Geometry: final body of the model. Coordinates: model frame, mm. A direction names the side the tool comes from. Give positions to 0.01 mm unless a question says otherwise; leave off trailing zeros. Loops run counter-clockwise (first coordinate to the right, second up) from the corner with the lowest first, then second, coordinate; pieces in that order, holes last.
Solid Edge part; units mm, degrees
sketch "Sketch1" plane through (0, 0, 0) normal (0, -1, 0) x (1, 0, 0)
  line L0 (-20.5, 32.9403) -> (20.5, 32.9403)
  line L1 (20.5, 32.9403) -> (20.5, 22.9403)
  line L2 (20.5, 22.9403) -> (28.5, 22.9403)
  line L3 (28.5, 22.9403) -> (28.5, 20.9403)
  line L4 (28.5, 20.9403) -> (20.5, 20.9403)
  line L5 (20.5, 20.9403) -> (20.5, -5.0597)
  line L6 (-20.5, -5.0597) -> (20.5, -5.0597)
  line L7 (-20.5, 20.9403) -> (-20.5, -5.0597)
  line L8 (-28.5, 20.9403) -> (-20.5, 20.9403)
  line L9 (-28.5, 22.9403) -> (-28.5, 20.9403)
  line L10 (-20.5, 22.9403) -> (-28.5, 22.9403)
  line L11 (-20.5, 32.9403) -> (-20.5, 22.9403)
  dimension "D1" = 20.5
  dimension "D2" = 20.5
  dimension "D3" = 28.5
  dimension "D4" = 20.5
  dimension "D5" = 28.5
extrude "Protrusion1" add sketch "Sketch1" along normal mid plane 21
sketch "Sketch2" plane through (0, 0, 32.9403) normal (0, 0, 1) x (1, 0, 0)
  circle A0 centre (-10.5, 0) radius 3
extrude "ProtrusiónExtruida_2" add sketch "Sketch2" along normal mid plane 4
Item 1: Section query D-D on y = 0. Return loops of the section in (x, z), plus the area to 3 significant figures.
Values follow:
outline: (-28.5, 20.94) - (-20.5, 20.94) - (-20.5, -5.06) - (20.5, -5.06) - (20.5, 20.94) - (28.5, 20.94) - (28.5, 22.94) - (20.5, 22.94) - (20.5, 32.94) - (-7.5, 32.94) - (-7.5, 34.94) - (-13.5, 34.94) - (-13.5, 32.94) - (-20.5, 32.94) - (-20.5, 22.94) - (-28.5, 22.94) - close
area: 1,600 mm2
Item 2: Section query A-A on x = -10.5. Return loops of the section in (y, z).
Values follow:
outline: (-10.5, -5.06) - (10.5, -5.06) - (10.5, 32.94) - (3, 32.94) - (3, 34.94) - (-3, 34.94) - (-3, 32.94) - (-10.5, 32.94) - close
Item 3: Set-up query: faces 1 (the face through (-12.9, 1.8, 33.9)), 2 (the face through (-25, 0, 20.94)), 3 (the face through (-20.5, 0, 28)), 4 (the face through (25, 0, 20.94)). Return all of +Z, -Z, +X, -X, +Y, -Y with unobstructed straight access to the full face (end or side cutting, diameter ignored); none if empty.
Values follow:
face 1: +Z
face 2: -Z, -X, +Y, -Y
face 3: +Z, -X, +Y, -Y
face 4: -Z, +X, +Y, -Y
Item 4: Section query C-C on z = 1. Return loops of the section in (x, y), plus the area to 3 significant figures.
Values follow:
outline: (-20.5, -10.5) - (20.5, -10.5) - (20.5, 10.5) - (-20.5, 10.5) - close
area: 861 mm2
Item 5: Ray query, probe 1 along Z at (x, y) = (9, -1.5); probe 2 along X at (y, z) = (-8, 2); probe 3 along Z at (x, y) = (24.5, -3). Return the intervals inside material, ascending.
Values follow:
probe 1: z = -5.06 to 32.94
probe 2: x = -20.5 to 20.5
probe 3: z = 20.94 to 22.94
Item 6: Section query B-B on y = 8. Return loops of the section in (x, z).
Values follow:
outline: (-28.5, 20.94) - (-20.5, 20.94) - (-20.5, -5.06) - (20.5, -5.06) - (20.5, 20.94) - (28.5, 20.94) - (28.5, 22.94) - (20.5, 22.94) - (20.5, 32.94) - (-20.5, 32.94) - (-20.5, 22.94) - (-28.5, 22.94) - close
Item 7: Pin query (flat end, axial travel): pin 1 (6.5 mm diameter, centred on x = 1.5, y = 1, fed in from +Z); pin 2 (6.5 mm diameter, centred on y = -3.5, z = 7, fed in from +X); pin 3 (9 mm diameter, centred on x = 26, y = 1, fed in from -Z). Return the tip coordinate at first contact, or that it passes through.
Values follow:
pin 1: stops at z = 32.94
pin 2: stops at x = 20.5
pin 3: stops at z = 20.94
